Autodesk Inventor part; units mm, degrees
ref_plane "YZ Plane" through (0, 0, 0) normal (1, 0, 0) x (0, 1, 0)
ref_plane "XZ Plane" through (0, 0, 0) normal (0, 1, 0) x (-1, 0, 0)
ref_plane "XY Plane" through (0, 0, 0) normal (0, 0, 1) x (1, 0, 0)
sketch "Sketch1" plane through (0, 0, 0) normal (0, 1, 0) x (-1, 0, 0)
  line L0 (98.0186, -101.2063) -> (-98.0186, -101.2063)
  line L1 (-98.0186, -101.2063) -> (-98.0186, 101.2063)
  line L2 (-98.0186, 101.2063) -> (98.0186, 101.2063)
  line L3 (98.0186, 101.2063) -> (98.0186, -101.2063)
  line L4 (98.0186, -101.2063) -> (-98.0186, 101.2063) construction
  line L5 (-98.0186, -101.2063) -> (98.0186, 101.2063) construction
  point P0 (0, 0)
  dimension "d0" = 196.0372
  dimension "d1" = 202.4126
extrude "Extrusion1" add sketch "Sketch1" along normal blind 3.175
sketch "Sketch2" plane through (0, 3.175, 0) normal (0, 1, 0) x (1, 0, 0)
  line L0 (98.0186, 101.2063) -> (-98.0186, 101.2063)
  line L1 (-98.0186, 101.2063) -> (-98.0186, -101.2063)
  line L2 (-98.0186, -101.2063) -> (98.0186, -101.2063)
  line L3 (98.0186, -101.2063) -> (98.0186, 101.2063)
  point P0 (0, 0)
  point P1 (-91.6686, 78.0923)
  point P2 (91.6686, 78.0923)
  point P3 (-91.6686, -78.0923)
  point P4 (91.6686, -78.0923)
  dimension "d4" = 23.114
  dimension "d5" = 23.114
  dimension "d6" = 6.35
  dimension "d7" = 6.35
hole "Hole1" at (-91.6686, 3.175, -78.0923) at (91.6686, 3.175, -78.0923) at (-91.6686, 3.175, 78.0923) at (91.6686, 3.175, 78.0923) direction (0, -1, 0) diameter 3.81 end through all
sketch "Sketch5" plane through (0, 3.175, 0) normal (0, 1, 0) x (1, 0, 0)
  line L0 (-98.0186, 101.2063) -> (-98.0186, -101.2063)
  line L1 (-98.0186, -101.2063) -> (98.0186, -101.2063)
  point P0 (0, 0)
  point P1 (-70.0786, -73.2663)
  point P2 (19.8374, -73.2663)
  point P3 (19.8374, 21.2217)
  point P4 (-70.0786, 21.2217)
  dimension "d44" = 27.94
  dimension "d45" = 27.94
  dimension "d46" = 89.916
  dimension "d47" = 94.488
hole "Hole4" at (-70.0786, 3.175, 73.2663) at (19.8374, 3.175, 73.2663) at (19.8374, 3.175, -21.2217) at (-70.0786, 3.175, -21.2217) direction (0, -1, 0) diameter 3.302 end through all
sketch "Sketch6" plane through (0, 3.175, 0) normal (0, 1, 0) x (1, 0, 0)
  circle A0 centre (-70.0786, -73.2663) radius 1.651
  circle A1 centre (19.8374, -73.2663) radius 1.651
  point P0 (0, 0)
  point P1 (-67.2846, -26.0223)
  point P2 (17.0434, -26.0223)
  dimension "d55" = 2.794
  dimension "d56" = 2.794
  dimension "d57" = 47.244
hole "Hole5" at (-67.2846, 3.175, 26.0223) at (17.0434, 3.175, 26.0223) direction (0, -1, 0) diameter 6.35 end through all
sketch "Sketch7" plane through (0, 3.175, 0) normal (0, 1, 0) x (1, 0, 0)
  circle A0 centre (-70.0786, 21.2217) radius 1.651
  line L0 (-48.2346, 13.3477) -> (-48.2346, 13.3477)
  line L1 (-41.8846, 6.9977) -> (-41.8846, -24.7523)
  line L2 (-48.2346, -31.1023) -> (-48.2346, -31.1023)
  line L3 (-54.5846, -24.7523) -> (-54.5846, 6.9977)
  arc A1 (-48.2346, 13.3477) -> (-54.5846, 6.9977) centre (-48.2346, 6.9977) ccw
  arc A2 (-41.8846, 6.9977) -> (-48.2346, 13.3477) centre (-48.2346, 6.9977) ccw
  arc A3 (-48.2346, -31.1023) -> (-41.8846, -24.7523) centre (-48.2346, -24.7523) ccw
  arc A4 (-54.5846, -24.7523) -> (-48.2346, -31.1023) centre (-48.2346, -24.7523) ccw
  point P0 (0, 0)
  dimension "d65" = 12.7
  dimension "d66" = 15.494
  dimension "d67" = 7.874
  dimension "d68" = 44.45
  dimension "d69" = 6.35
extrude "Extrusion2" cut sketch "Sketch7" against normal blind 25.4 contours L1 A3 A4 L3 A1 A2
sketch "Sketch8" plane through (0, 3.175, 0) normal (0, 1, 0) x (1, 0, 0)
  line L0 (-98.0186, -101.2063) -> (98.0186, -101.2063)
  line L1 (98.0186, -101.2063) -> (98.0186, 101.2063)
  point P0 (0, 0)
  point P1 (76.4286, -31.3563)
  dimension "d72" = 21.59
  dimension "d73" = 69.85
hole "Hole6" at (76.4286, 3.175, 31.3563) direction (0, -1, 0) diameter 6.985 end through all
sketch "Sketch9" plane through (0, 3.175, 0) normal (0, 1, 0) x (1, 0, 0)
  circle A0 centre (76.4286, -31.3563) radius 3.4925
  point P0 (0, 0)
  point P1 (69.4436, -14.2113)
  point P2 (69.4436, -48.5013)
  dimension "d81" = 6.985
  dimension "d82" = 17.145
  dimension "d83" = 17.145
hole "Hole7" at (69.4436, 3.175, 14.2113) at (69.4436, 3.175, 48.5013) direction (0, -1, 0) diameter 3.302 end through all
sketch "Sketch10" plane through (0, 3.175, 0) normal (0, 1, 0) x (1, 0, 0)
  line L0 (98.0186, 101.2063) -> (-98.0186, 101.2063)
  line L1 (98.0186, -101.2063) -> (98.0186, 101.2063)
  line L2 (0, 56.7563) -> (0, 92.8243)
  point P0 (0, 0)
  point P1 (-52.8574, 92.8243)
  point P2 (-43.9674, 56.7563)
  point P3 (52.8574, 92.8243)
  point P4 (43.9674, 56.7563)
  dimension "d91" = 52.8574
  dimension "d92" = 8.382
  dimension "d93" = 36.068
  dimension "d94" = 8.89
hole "Hole8" at (-52.8574, 3.175, -92.8243) at (-43.9674, 3.175, -56.7563) at (52.8574, 3.175, -92.8243) at (43.9674, 3.175, -56.7563) direction (0, -1, 0) diameter 3.302 end through all
sketch "Sketch11" plane through (0, 3.175, 0) normal (0, 1, 0) x (1, 0, 0)
  circle A0 centre (76.4286, -31.3563) radius 3.4925
  line L0 (98.0186, 101.2063) -> (-98.0186, 101.2063)
  point P0 (0, 0)
  point P1 (76.4286, 6.5913)
  point P2 (76.4286, 63.1063)
  dimension "d103" = 56.515
  dimension "d111" = 38.1
hole "Hole9" at (76.4286, 3.175, -6.5913) at (76.4286, 3.175, -63.1063) direction (0, -1, 0) diameter 3.302 end through all
sketch "Sketch12" plane through (0, 3.175, 0) normal (0, 1, 0) x (1, 0, 0)
  line L0 (98.0186, 101.2063) -> (-98.0186, 101.2063)
  line L1 (-98.0186, 101.2063) -> (-98.0186, -101.2063)
  line L2 (-98.0186, -101.2063) -> (98.0186, -101.2063)
  line L3 (98.0186, -101.2063) -> (98.0186, 101.2063)
  point P0 (0, 0)
  point P1 (-78.9686, -93.5863)
  point P2 (78.9686, -93.5863)
  point P3 (78.9686, 93.5863)
  point P4 (-78.9686, 93.5863)
  dimension "d112" = 7.62
  dimension "d113" = 19.05
  dimension "d114" = 7.62
  dimension "d115" = 19.05
hole "Hole10" at (-78.9686, 3.175, 93.5863) at (78.9686, 3.175, 93.5863) at (78.9686, 3.175, -93.5863) at (-78.9686, 3.175, -93.5863) direction (0, -1, 0) diameter 3.302 end through all
properties part number "SwarmieTopPlate"
Read the model definition and answer for the solid it produces. Units are mm, in the model's axes. A direction names the side the tool comes from. Give positions to 0.01 mm unless a question says otherwise; leave off trailing zeros.
(1) Find section A-A (y = 1.95). Give the number of separate pieces and of enclosed holes in the cut face, plus the area to 3 significant figures.
(2) Straight lines are drawn through the part: L1, parallel to X at y = 2.6, z = -57; L2, parallel to Z at x = -45, y = 2.9; L3, parallel to X at y = 1.8, z = 9.5. For each, find the intervals that lie inside material, in ascending order.
(3) Given pin 1 (4 mm diameter, centred on x = 19.84, z = -21.22, fed in from +Y) (3 decimals), flat-ended and moving along its own axis, determine where the tip first touches the part or whether it passes through.
(4) For faces 1 (the flat face through (1, 0, 1)), 2 (the cylindrical face through (-48.4, 1.6, 31.1)), determine the directions among +Z, -Z, +X, -X, +Y, -Y from which every point of the face is accessible in a straight line to the end or side of a thin tool.
Result sheet:
1. separate pieces: 1
1. enclosed holes: 24
1. area: 38,900 mm2
2. L1: x = -98.02 to -45.6, -42.33 to 42.33, 45.6 to 98.02
2. L2: z = -101.21 to -58.04, -55.47 to -12.46, 30.22 to 101.21
2. L3: x = -98.02 to -54.58, -41.88 to 98.02
3. pin 1: stops at y = 3.175
4. face 1: +Z, -Z, +X, -X, -Y
4. face 2: +Y, -Y
